Input: part model. Units: mm. Frame: model coordinates. Coordinates: 2 decimals unless noted, no trailing zeros. Write each loop counter-clockwise with the first axis right and the second up, starting at its lowest first coordinate (ties: lowest second). Pieces come first, ordered by that corner, then holes.
1) Pin query (flat end, axial travel): pin 1 Ø5.5 at (x, y) = (43.5, 43.5) entering from +Z; pin 2 Ø1 at (x, z) = (23, -2) entering from +Y. Return the tip coordinate at first contact, or that it passes through.
2) Draft query along Y for faces 1 (the flat face through (14.7, 56.4, -0.5)), 2 (the flat face through (87, 14, 0)), 3 (the cylindrical face through (40.003, 13.654, -0.035)). Return one class per face: pulls with the +Y half, pulls with the -Y half, needs draft (parallel to the pull), parting line crosses it, or undercut.
3) Line query: L1, parallel to Y at x = 43.5, z = -0.35; L2, parallel to X at y = 29, z = 1.3; L3, parallel to Y at x = 73.5, z = -2.2. Output: solid intervals per line, ascending.
4) Section query A-A (y = 13.5). Output: boundary loops of the cut face in (x, z).
5) Section query C-C (z = -0.15). Output: boundary loops of the cut face in (x, y).
from build123d import *

# Parameters (mm, degrees)
SKETCH1_R           = 3.5
BOSS_EXTRUDE1_DEPTH = 2.5
FILLET1_R           = 1


with BuildPart() as part:
    # Sketch1 → Boss-Extrude1 (new body, symmetric)
    with BuildSketch(Plane.XY):
        Polygon((0, 0), (0, 27), (30, 87), (57, 87), (87, 27), (87, 0), align=None)
        with Locations((13.5, 13.5)):
            Circle(SKETCH1_R, mode=Mode.SUBTRACT)
        with Locations((43.5, 13.5)):
            Circle(SKETCH1_R, mode=Mode.SUBTRACT)
        with Locations((73.5, 13.5)):
            Circle(SKETCH1_R, mode=Mode.SUBTRACT)
        with Locations((43.5, 43.5)):
            Circle(SKETCH1_R, mode=Mode.SUBTRACT)
        with Locations((43.5, 73.5)):
            Circle(SKETCH1_R, mode=Mode.SUBTRACT)
    extrude(amount=BOSS_EXTRUDE1_DEPTH, both=True)

    # Fillet1
    fillet1_edges = [part.edges().sort_by_distance(p)[0] for p in [
        (72, 57, 2.5),
        (0, 0, 0),
        (0, 27, 0),
        (30, 87, 0),
        (57, 87, 0),
        (87, 27, 0),
        (87, 0, 0),
        (43.5, 87, 2.5),
        (15, 57, 2.5),
        (0, 13.5, 2.5),
        (43.5, 0, 2.5),
        (87, 13.5, 2.5),
    ]]
    fillet(fillet1_edges, radius=FILLET1_R)


solid = part.part
Answer:
1. pin 1: passes through
1. pin 2: stops at y = 74
2. face 1: pulls with the +Y half
2. face 2: needs draft
2. face 3: undercut
3. L1: y = 0 to 10, 17 to 40, 47 to 70, 77 to 87
3. L2: x = 1 to 86
3. L3: y = 0 to 10, 17 to 54
4. outline: (0, -2.5) - (10, -2.5) - (10, 2.5) - (1, 2.5) arc R1 ccw to (0, 1.5) - close; (17, -2.5) - (40, -2.5) - (40, 2.5) - (17, 2.5) - close; (47, -2.5) - (70, -2.5) - (70, 2.5) - (47, 2.5) - close; (77, -2.5) - (87, -2.5) - (87, 1.5) arc R1 ccw to (86, 2.5) - (77, 2.5) - close
5. outline: (0, 1) arc R1 ccw to (1, 0) - (86, 0) arc R1 ccw to (87, 1) - (87, 26.76) arc R1 ccw to (86.89, 27.21) - (57.28, 86.45) arc R1 ccw to (56.38, 87) - (30.62, 87) arc R1 ccw to (29.72, 86.45) - (0.11, 27.21) arc R1 ccw to (0, 26.76) - close; hole circle Ø7 at (13.5, 13.5); hole circle Ø7 at (43.5, 13.5); hole circle Ø7 at (43.5, 43.5); hole circle Ø7 at (43.5, 73.5); hole circle Ø7 at (73.5, 13.5)
